Design review of the part built by this model. Coordinates are the model's own, in mm. A direction names the side the tool comes from. Coordinates: 2 decimals unless noted, no trailing zeros. Write each loop counter-clockwise with the first axis right and the second up, starting at its lowest first coordinate (ties: lowest second). Pieces come first, ordered by that corner, then holes. Notation, with made-up numbers: (89.25, 75) - (98.25, 75) arc R30 cw to (98.25, 111) - close; hole circle Ø9 at (3.5, 89.25). An arc over 180 degrees is marked (long way). Use a Markdown table: item, result.
from build123d import *

# Parameters (mm, degrees)
F0_W     = 55
F0_H     = 55
F0_W_2   = 50
F0_H_2   = 50
F1_DEPTH = 75
F3_D     = 8.8
F4_W     = 50
F4_H     = 50
F4_W_2   = 45
F4_H_2   = 45
F5_DEPTH = 275
F7_D     = 8.8


with BuildPart() as f1:
    # F0 (on Top) → F1 (new body)
    with BuildSketch(Plane.XY):
        Rectangle(F0_W, F0_H)
        Rectangle(F0_W_2, F0_H_2, mode=Mode.SUBTRACT)
    extrude(amount=F1_DEPTH)

    # F3 (through all)
    with Locations(Plane(origin=(-27.5, 0, 0), x_dir=(0, -1, 0), z_dir=(-1, 0, 0))):
        with Locations((0, 37.5)):
            Hole(F3_D / 2)

    # F4 (on face) → F5 (join)
    with BuildSketch(Plane.XZ.offset(27.5)):
        with Locations((0, 37.5)):
            Rectangle(F4_W, F4_H)
        with Locations((0, 37.5)):
            Rectangle(F4_W_2, F4_H_2, mode=Mode.SUBTRACT)
    extrude(amount=F5_DEPTH)

    # F7 (through all)
    with Locations(Plane.XY.offset(62.5)):
        with Locations((0, -277.5)):
            Hole(F7_D / 2)


solid = f1.part
(1) Take a section at B-B on z = 37.5. Write out the cut boundary in (x, y).
Determined:
| item | result |
|---|---|
| outline | (-27.5, -27.5) - (-25, -27.5) - (-25, -302.5) - (-22.5, -302.5) - (-22.5, -27.5) - (22.5, -27.5) - (22.5, -302.5) - (25, -302.5) - (25, -27.5) - (27.5, -27.5) - (27.5, -4.4) - (25, -4.4) - (25, -25) - (-25, -25) - (-25, -4.4) - (-27.5, -4.4) - close; (-27.5, 4.4) - (-25, 4.4) - (-25, 25) - (25, 25) - (25, 4.4) - (27.5, 4.4) - (27.5, 27.5) - (-27.5, 27.5) - close |
(2) Take a section at C-C on x = 0. Write out the cut boundary in (y, z).
Determined:
| item | result |
|---|---|
| outline | (-302.5, 12.5) - (-281.9, 12.5) - (-281.9, 15) - (-302.5, 15) - close; (-302.5, 60) - (-281.9, 60) - (-281.9, 62.5) - (-302.5, 62.5) - close; (-273.1, 12.5) - (-27.5, 12.5) - (-27.5, 0) - (-25, 0) - (-25, 75) - (-27.5, 75) - (-27.5, 62.5) - (-273.1, 62.5) - (-273.1, 60) - (-27.5, 60) - (-27.5, 15) - (-273.1, 15) - close; (25, 0) - (27.5, 0) - (27.5, 75) - (25, 75) - close |
(3) For pin 1 (1.5 mm diameter, centred on y = -74.5, z = 21.5, fed in from +X); pin 2 (2 mm diameter, centred on x = 18.5, z = 31.5, fed in from -Y); pin 3 (22.5 mm diameter, centred on x = 3.5, y = -172, fed in from +Z), all flat-tipped, find the tip position at first contact; note any pin that passes through.
Determined:
| item | result |
|---|---|
| pin 1 | x = 25 |
| pin 2 | y = -27.5 |
| pin 3 | z = 62.5 |
(4) Machinability: for faces 1 (the flat face through (0, -163, 62.5)), 2 (the flat face through (-25, -163, 37)), 3 (the flat face through (0, -27.5, 37)), 4 (the cylindrical face through (0.573, -273.137, 13.733)), 5 (the flat face through (-27.5, -6, 37)), which of the approach directions +Z, -Z, +X, -X, +Y, -Y give a long, thin tool a straight path to every point of the face, cutting with its end or side? Answer none if there is none.
Determined:
| item | result |
|---|---|
| face 1 | +Z, +X, -X, -Y |
| face 2 | +Z, -Z, -X, -Y |
| face 3 | -Y |
| face 4 | +Z, -Z |
| face 5 | +Z, -Z, -X, +Y, -Y |
(5) Take a section at D-D on z = 21. Write out the cut boundary in (x, y).
Determined:
| item | result |
|---|---|
| outline | (-27.5, -27.5) - (-25, -27.5) - (-25, -302.5) - (-22.5, -302.5) - (-22.5, -27.5) - (22.5, -27.5) - (22.5, -302.5) - (25, -302.5) - (25, -27.5) - (27.5, -27.5) - (27.5, 27.5) - (-27.5, 27.5) - close; hole (-25, -25) - (25, -25) - (25, 25) - (-25, 25) - close |
(6) Draft analysis for pull direction Y (two halves, no side actions). For faces 6 (the flat face through (0, -163, 12.5)), 7 (the flat face through (-25, -6, 37)), 8 (the flat face through (0, 27.5, 37)), 9 (the flat face through (0, -25, 37)), state which applies: +Y half, -Y half, draft (parallel to the pull), parting line (faces both ways), or undercut.
Determined:
| item | result |
|---|---|
| face 6 | draft |
| face 7 | undercut |
| face 8 | +Y half |
| face 9 | undercut |
(7) For L1, parallel to Y at x = 0, z = 61; L2, parallel to X at y = -11.5, z = 65.5, list the stretches that pass through material, from the lowest coordinate up. Write a range as from..to.
Determined:
| item | result |
|---|---|
| L1 | -302.5..-281.9, -273.1..-25, 25..27.5 |
| L2 | -27.5..-25, 25..27.5 |
(8) Take a section at A-A on y = -277.5. Write out the cut boundary in (x, z).
Determined:
| item | result |
|---|---|
| outline | (-25, 12.5) - (-4.4, 12.5) - (-4.4, 15) - (-22.5, 15) - (-22.5, 60) - (-4.4, 60) - (-4.4, 62.5) - (-25, 62.5) - close; (4.4, 12.5) - (25, 12.5) - (25, 62.5) - (4.4, 62.5) - (4.4, 60) - (22.5, 60) - (22.5, 15) - (4.4, 15) - close |
